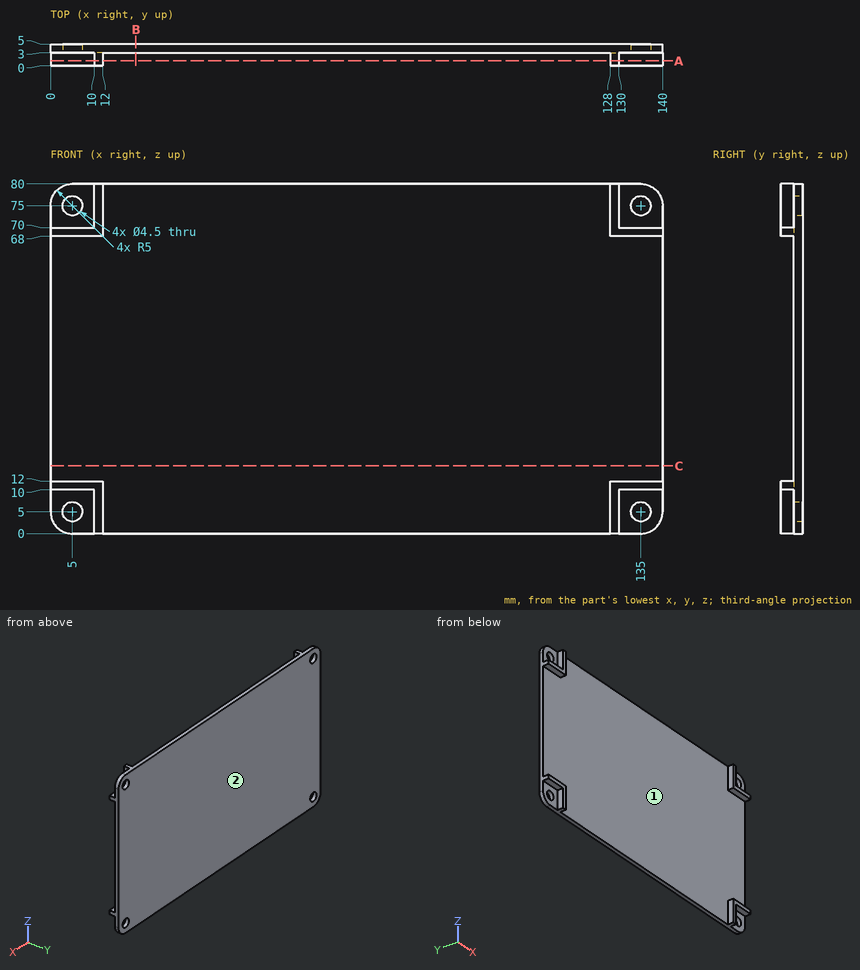
Study the drawing (mm; zero at the part's minimum x, y, z) and answer. Round coordinates to 2 decimals unless told otherwise and drop trailing zeros. Write each loop counter-clockwise with the first axis right and the second up, starting at its lowest first coordinate (ties: lowest second). Pieces come first, ordered by that corner, then holes.
1) A cutting plane is placed at C-C on z = 15.5. Determine the outline of the cut face in (x, y).
2) Consider probe 1 along X at (y, z) = (4.1, 5); probe 2 along Y at (x, z) = (38.5, 61.5); probe 3 along X at (y, z) = (2, 8.5). Determine where each line is inside the solid, lowest interval first.
3) A cutting plane is placed at B-B on x = 19.5. Determine the outline of the cut face in (y, z).
4) Flat-ended cylindrical pins translate along their axes: P1, Ø2.5, axis at x = 5.5, y = 1.5, coming from the -Z side; P2, Ø2.5, axis at x = 135, z = 5, coming from the +Y side (3 decimals); P3, Ø3, axis at x = 6.5, z = 74, coming from the -Y side; P4, Ø2.5, axis at x = 5, y = 1.5, coming from the +Z side. Find the tip coordinate at first contact, or state that the pin passes through.
5) A cutting plane is placed at A-A on y = 1.15. Determine the outline of the cut face in (x, z).
6) Determine the mould class of the marked faces 1 and 2 for opening direction Z: pulls with the +Z half, pulls with the -Z half, needs draft (parallel to the pull), parting line crosses it, or undercut.
Entries:
1. outline: (0, 3) - (140, 3) - (140, 5) - (0, 5) - close
2. probe 1: x = 0 to 2.75, 7.25 to 132.75, 137.25 to 140
2. probe 2: y = 3 to 5
2. probe 3: x = 10 to 12, 128 to 130
3. outline: (3, 0) - (5, 0) - (5, 80) - (3, 80) - close
4. P1: stops at z = 10
4. P2: passes through
4. P3: stops at y = 3
4. P4: stops at z = 70
5. outline: (0, 10) - (10, 10) - (10, 0) - (12, 0) - (12, 12) - (0, 12) - close; (0, 68) - (12, 68) - (12, 80) - (10, 80) - (10, 70) - (0, 70) - close; (128, 0) - (130, 0) - (130, 10) - (140, 10) - (140, 12) - (128, 12) - close; (128, 68) - (140, 68) - (140, 70) - (130, 70) - (130, 80) - (128, 80) - close
6. face 1: undercut
6. face 2: needs draft
